Could you check a few things on this model? Use its own coordinates, in mm. A direction names the side the tool comes from. Coordinates: 2 decimals unless noted, no trailing zeros. Loops run counter-clockwise (first coordinate to the right, second up) from the corner with the lowest first, then second, coordinate; pieces in that order, holes last.
Autodesk Inventor part; units mm, degrees
ref_plane "Work Plane1" through (33.575, 0, 0) normal (0, 0, -1) x (1, 0, 0)
ref_plane "YZ Plane" through (0, 0, 0) normal (1, 0, 0) x (0, 1, 0)
ref_plane "XZ Plane" through (0, 0, 0) normal (0, 1, 0) x (-1, 0, 0)
sketch "스케치1" plane through (0, 0, 0) normal (0, 0, 1) x (1, 0, 0)
  line L0 (0, 0) -> (10, 0)
  line L1 (10, 0) -> (10, 1.5)
  line L2 (10, 1.5) -> (2.65, 1.5)
  line L3 (2.65, 1.5) -> (2.3433, 1.1933)
  line L4 (2.3433, 1.1933) -> (1.9567, 1.1933)
  line L5 (1.9567, 1.1933) -> (0.4, 2.75)
  line L6 (0.4, 2.75) -> (0, 2.75)
  line L7 (0, 2.75) -> (0, 0)
  line L8 (2.65, 1.5) -> (1.65, 1.5) construction
  line L9 (-2, 0) -> (12, 0)
  line L10 (0, 3.3) -> (0, -0.55)
  dimension "d0" = 10
  dimension "d1" = 45
  dimension "d2" = 0.3067
  dimension "d4" = 1.65
  dimension "d5" = 2.3866
  dimension "d6" = 3
  dimension "d7" = 5.5
revolve "본체" add sketch "스케치1" angle 360 about axis through (0, 0, 0) along (1, 0, 0)
sketch "스케치2" plane through (0, 0, 0) normal (-1, 0, 0) x (0, 0, 1)
  line L0 (2.75, -0.4) -> (-2.75, -0.4)
  line L1 (-2.75, -0.4) -> (-2.75, 0.4)
  line L2 (-2.75, 0.4) -> (2.75, 0.4)
  line L3 (2.75, 0.4) -> (2.75, -0.4)
  line L4 (0, 0.4) -> (0, -0.4) construction
  line L5 (-2.75, 0) -> (2.75, 0) construction
  line L6 (0, 2.75) -> (0, 0)
  dimension "d15" = 0.8
  dimension "d16" = 5.5
extrude "슬롯" cut sketch "스케치2" against normal blind 0.6
thread "스레드"
chamfer "모따기1" distance 0.3067 distance2 0.1534 1 edges at (10, -1.5, 0) measured on face at (10, -0.5495, 0.6466)
ref_plane "Work Plane1" through (33.575, 0, 0) normal (0, 0, -1) x (1, 0, 0)
equation "\"d15\" = SBR"
equation "\"d16\" = KOD"
equation "\"d8\" = STI"
equation "\"d12\" = -0.5 * SPD + 0.5 * GD"
equation "\"d13\" = 0.5 * GAL"
equation "\"d1\" = 0.5 * SEWI"
equation "\"d2\" = GAL"
equation "\"d4\" = KOH"
equation "\"d5\" = BDM"
equation "\"d6\" = GD"
equation "\"d7\" = KOD"
equation "\"NLG\" = 6"
equation "\"GAL\" = 0.61345 * PTC"
equation "\"GEL\" = 3.35"
equation "\"KOH\" = 1.65"
equation "\"KOD\" = 5.5"
equation "\"SEWI\" = 90deg"
equation "\"BDM\" = NND - 1.2269 * PTC"
equation "\"GD\" = NND"
equation "\"SBR\" = 0.8"
equation "\"STI\" = 0.6"
equation "\"SPD\" = NND - 1.2269 * PTC"
equation "\"GUL\" = 0.61345 * PTC"
equation "\"PTC\" = 0.5"
equation "\"EPV\" = 3.15"
equation "\"THREADDIA\" = 3"
equation "\"TOA\" = 30deg"
equation "\"NND\" = 3"
equation "\"GD1\" = THREADDIA - 1.2269 * PTC"
properties part number "KS B 1021 - M 3 x 6(1)" material "강철, 연강"
(1) Imagine slicing it at A-A, the plane z = 0. Write out the boundary of the cut face in (x, y), and give its area (3 significant figures).
Answers:
outline: (0, -2.75) - (0.4, -2.75) - (1.96, -1.19) - (2.34, -1.19) - (2.65, -1.5) - (9.85, -1.5) - (10, -1.19) - (10, 1.19) - (9.85, 1.5) - (2.65, 1.5) - (2.34, 1.19) - (1.96, 1.19) - (0.4, 2.75) - (0, 2.75) - (0, 0.4) - (0.6, 0.4) - (0.6, -0.4) - (0, -0.4) - close
area: 31.6 mm2
(2) We'd pull the mould along Y, two halves only. Please class faces 3 (the face through (10, 0, 0)), 4 (the face through (0.6, 0, 0)), 5 (the face through (2.147, -0.88, -0.806)): +Y half, -Y half, draft (parallel to the pull), parting line (faces both ways), or undercut.
Answers:
face 3: draft
face 4: undercut
face 5: parting line
(3) I need wall thicknesses on probe 1 along X at (y, z) = (1, -0.75); probe 2 along Z at (x, y) = (4, 0.1); probe 3 along X at (y, z) = (1.4, -0.3). Which ranges of each line are inside material? Lowest first, please.
Answers:
probe 1: x = 0 to 1.9, 2.4 to 9.97
probe 2: z = -1.5 to 1.5
probe 3: x = 0 to 1.72, 2.58 to 9.88
(4) Imagine slicing it at C-C, the plane x = 5. Write out the boundary of the cut face in (y, z).
Answers:
outline: circle Ø3 at (0, 0)
(5) Imagine slicing it at B-B, the plane y = 0. Write out the boundary of the cut face in (x, z).
Answers:
outline: (0.6, -2.55) - (1.96, -1.19) - (2.34, -1.19) - (2.65, -1.5) - (9.85, -1.5) - (10, -1.19) - (10, 1.19) - (9.85, 1.5) - (2.65, 1.5) - (2.34, 1.19) - (1.96, 1.19) - (0.6, 2.55) - close
(6) For pin 1 (3 mm diameter, centred on x = 8.5, y = -1.5, fed in from -Z); pin 2 (0.7 mm diameter, centred on x = 0, z = 1.5, fed in from -Y); pin 3 (0.7 mm diameter, centred on x = 0.5, z = 1, fed in from +Y), each with a flat end and sliding along its axis, tell me the tip position at first contact or that it passes through.
Answers:
pin 1: stops at z = -1.5
pin 2: stops at y = -2.5
pin 3: stops at y = 2.67
(7) Which directions (+Z, -Z, +X, -X, +Y, -Y) give clear straight access to the entire face, cutting with the end or side of a thin tool? Please do faces 1 (the face through (6.2, -1.5, -0.07)), 2 (the face through (0, 1, 0)).
Answers:
face 1: +X
face 2: +Z, -Z, -X, +Y, -Y
